Check sheet for the modelled part. Datum: model origin and axes. Units: mm. Face numbers are marked on the shaded views. A direction names the side the tool comes from. Coordinates: 2 decimals unless noted, no trailing zeros. Loops run counter-clockwise (first coordinate to the right, second up) from the corner with the lowest first, then second, coordinate; pieces in that order, holes last. Notation, with made-up numbers: (10, 84) -> (52, 84) arc R9 cw to (52, 89) -> close; hole circle Ø11 at (42.25, -25). An arc over 180 degrees is marked (long way). Use CSV: the item, a comma, the result in double quotes. Start each with the question number.
1. Sectioned sample at D-D, the plane z = 0. Record the cut outline in (x, y), and give its area (3 significant figures).
2. Gauge pin test, flat ends, axial feed: pin 1 (2.5 mm diameter, centred on y = 6.5, z = 0, fed in from +X); pin 2 (1 mm diameter, centred on x = -13.5, z = 23.5, fed in from +Y); pin 3 (4.5 mm diameter, centred on y = 7.5, z = 1, fed in from -X); pin 4 (1.5 mm diameter, centred on x = 0, z = -27.46, fed in from +Y). Record the tip position at first contact, or that the pin passes through.
3. Sectioned sample at C-C, the plane z = -27.46. Record the cut outline in (x, y), and give its area (3 significant figures).
4. Set-up check for the marked faces 1, 2, 3, 4 and 5: record each of +Z, -Z, +X, -X, +Y, -Y from which the full face is reachable in a straight line by a thin tool's end or side.
5. Sectioned sample at B-B, the plane y = 8. Record the cut outline in (x, z).
6. Thickness scan on L1, parallel to Z at x = 0, y = 1.1; L2, parallel to X at y = 5.5, z = -3.5; L3, parallel to Z at x = -6.5, y = 7.25. Record the ranges inside material, lowest first.
7. Sectioned sample at A-A, the plane x = 0. Record the cut outline in (y, z), and give its area (3 significant figures).
```python
from build123d import *

# Parameters (mm, degrees)
SKETCH1_R           = 30
BOSS_EXTRUDE1_DEPTH = 1.64
SKETCH2_R           = 1.27
CUT_EXTRUDE1_DEPTH  = 2.64
SKETCH3_W           = 19.304
SKETCH3_H           = 10
BOSS_EXTRUDE2_DEPTH = 8.6


with BuildPart() as part:
    # Sketch1 → Boss-Extrude1 (new body)
    with BuildSketch(Plane(origin=(0, 0, 0), x_dir=(1, 0, 0), z_dir=(0, 1, 0))):
        Circle(SKETCH1_R)
    extrude(amount=BOSS_EXTRUDE1_DEPTH)

    # Sketch2 → Cut-Extrude1 (cut, through all)
    with BuildSketch(Plane(origin=(0, 1.64, 0), x_dir=(1, 0, 0), z_dir=(0, 1, 0))):
        with Locations((0, 27.46)):
            Circle(SKETCH2_R)
        with Locations((0, -27.46)):
            Circle(SKETCH2_R)
    extrude(amount=-CUT_EXTRUDE1_DEPTH, mode=Mode.SUBTRACT)

    # Sketch3 → Boss-Extrude2 (add)
    with BuildSketch(Plane(origin=(0, 1.64, 0), x_dir=(1, 0, 0), z_dir=(0, 1, 0))):
        with Locations((-13.948, 0)):
            Rectangle(SKETCH3_W, SKETCH3_H)
        with Locations((13.948, 0)):
            Rectangle(SKETCH3_W, SKETCH3_H)
    extrude(amount=BOSS_EXTRUDE2_DEPTH)


solid = part.part
```
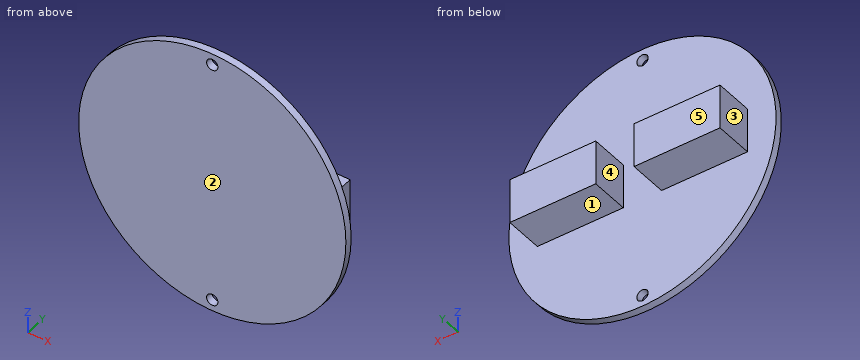
Completed:
1,outline,"(-30, 0) -> (30, 0) -> (30, 1.64) -> (23.6, 1.64) -> (23.6, 10.24) -> (4.3, 10.24) -> (4.3, 1.64) -> (-4.3, 1.64) -> (-4.3, 10.24) -> (-23.6, 10.24) -> (-23.6, 1.64) -> (-30, 1.64) -> close"
1,area,"430 mm²"
2,pin 1,"x = 23.6"
2,pin 2,"y = 1.64"
2,pin 3,"x = -23.6"
2,pin 4,"through"
3,outline,"(-12.08, 0) -> (-1.27, 0) -> (-1.27, 1.64) -> (-12.08, 1.64) -> close; (1.27, 0) -> (12.08, 0) -> (12.08, 1.64) -> (1.27, 1.64) -> close"
3,area,"35.5 mm²"
4,face 1,"-Z, +X, -X, +Y"
4,face 2,"+Z, -Z, +X, -X, -Y"
4,face 3,"+Z, -Z, -X, +Y"
4,face 4,"+Z, -Z, +Y"
4,face 5,"+Z, -Z, +X, -X, +Y"
5,outline,"(-23.6, -5) -> (-4.3, -5) -> (-4.3, 5) -> (-23.6, 5) -> close; (4.3, -5) -> (23.6, -5) -> (23.6, 5) -> (4.3, 5) -> close"
6,L1,"-30 to -28.73, -26.19 to 26.19, 28.73 to 30"
6,L2,"-23.6 to -4.3, 4.3 to 23.6"
6,L3,"-5 to 5"
7,outline,"(0, -30) -> (1.64, -30) -> (1.64, -28.73) -> (0, -28.73) -> close; (0, -26.19) -> (1.64, -26.19) -> (1.64, 26.19) -> (0, 26.19) -> close; (0, 28.73) -> (1.64, 28.73) -> (1.64, 30) -> (0, 30) -> close"
7,area,"90.1 mm²"
